```python
from build123d import *

# Parameters (mm, degrees)
F1_DEPTH = 3
F2_SIZE  = 2.99999
F4_D     = 10
F4_DEPTH = 9
F4_TIP   = 3.0043030951


# Not quite as in the source:
# - a fillet or chamfer is up to 0.001 mm smaller than in the source, because OpenCascade refuses the exact size


with BuildPart() as f1:
    # F0 (on Front) → F1 (new body)
    with BuildSketch(Plane.XZ):
        with BuildLine():
            Line((0, 90), (0, 0))
            Line((0, 0), (90, 0))
            Line((90, 0), (90, 45))
            ThreePointArc((90, 45), (58.1801948466, 58.1801948466), (45, 90))
            Line((45, 90), (0, 90))
        make_face()
    extrude(amount=F1_DEPTH)

    # F2 (size 3 in the source; OpenCascade refuses exactly that, so slightly less here)
    f2_edges = [f1.edges().sort_by_distance(p)[0] for p in [
        (22.5, -3, 90),
        (0, -3, 45),
        (45, -3, 0),
        (90, -3, 22.5),
        (58.180195, -3, 58.180195),
    ]]
    chamfer(f2_edges, length=F2_SIZE)

    # F4
    with Locations(Plane.XZ.offset(3)):
        with Locations((12, 78), (33.093841732, 78), (78, 33.093841732), (78, 12)):
            Hole(F4_D / 2, depth=F4_DEPTH)
            with Locations((0, 0, -(F4_DEPTH + F4_TIP / 2))):  # 118° drill point
                Cone(0, F4_D / 2, F4_TIP, mode=Mode.SUBTRACT)


solid = f1.part
```
The listing builds one solid part. Answer for the finished solid, in the listing's coordinates (mm). Coordinates: 2 decimals unless noted, no trailing zeros. Loops run counter-clockwise (first coordinate to the right, second up) from the corner with the lowest first, then second, coordinate; pieces in that order, holes last. Notation, with made-up numbers: M 30.5,-15 L 40.5,-15 A15 ccw 40.5,10 Z; hole C 39.25,44.25 d11. An arc over 180 degrees is marked long. Answer as a JSON object with one key per item and string values. Group by question number.
Item 1: Consider L1, parallel to Z at x = 81.5, y = -0.15; L2, parallel to X at y = -1.3, z = 79; L3, parallel to Z at x = 78, y = -1.75. Determine where each line is inside the solid, lowest interval first.
Item 2: This flat-tipped pin is pushed along its axis until it touches: P1, Ø1.5, axis at y = -2, z = 18, coming from the -X side. Where does it stop, or does it pass through?
Item 3: Section D-D (x = 79.5) is taken. Give the number of separate pieces and of enclosed holes in the cut face, and give its area (3 significant figures).
Item 4: Determine the mould class of faces 1 (the face through (73.23, -1.48, 13.5)), 2 (the face through (75.3, -1.5, 37.3)), 3 (the face through (88, -2, 22)), 4 (the face through (35, -3, 36)) for opening direction X: +X half, -X half, draft (parallel to the pull), parting line (faces both ways), or undercut.
Item 5: Section C-C (y = -1.75) is taken. Write down the section's boundary in (x, z).
Solved:
{
 "1": {"L1": "z = 0.15 to 8.43, 15.57 to 29.52, 36.66 to 45.66", "L2": "x = 1.3 to 7.1, 16.9 to 28.19, 37.99 to 45.03", "L3": "z = 1.75 to 7, 17 to 28.09, 38.09 to 44.82"},
 "2": {"P1": "stops at x = 1.25"},
 "3": {"separate pieces": "3", "enclosed holes": "0", "area": "72.4 mm2"},
 "4": {"face 1": "undercut", "face 2": "undercut", "face 3": "+X half", "face 4": "draft"},
 "5": {"outline": "M 1.75,1.75 L 88.25,1.75 L 88.25,43.28 A46.75 cw 43.28,88.25 L 1.75,88.25 Z; hole C 12,78 d10; hole C 33.09,78 d10; hole C 78,12 d10; hole C 78,33.09 d10"}
}
